```python
from build123d import *

# Parameters (mm, degrees)
SKETCH1_W                = 762
SKETCH1_H                = 457.2
BOSS_EXTRUDE1_DEPTH      = 177.8
SKETCH2_W                = 749.3
SKETCH2_H                = 444.5
CUT_EXTRUDE1_DEPTH       = 171.45
SKETCH4_W                = 758.825
SKETCH4_H                = 454.025
SKETCH4_W_2              = 752.475
SKETCH4_H_2              = 447.675
CUT_EXTRUDE3_DEPTH       = 3.175
SKETCH5_W                = 762
SKETCH5_H                = 12.7
BOSS_EXTRUDE2_DEPTH      = 177.8
BOSS_EXTRUDE2_DEPTH_BACK = 38.1
SKETCH7_R                = 6.35
BOSS_EXTRUDE3_DEPTH      = 762
SKETCH8_W                = 12.7
SKETCH8_H                = 38.1
CUT_EXTRUDE4_DEPTH       = 202.692


with BuildPart() as part:
    # Sketch1 → Boss-Extrude1 (new body)
    with BuildSketch(Plane(origin=(0, 0, 0), x_dir=(1, 0, 0), z_dir=(0, 1, 0))):
        Rectangle(SKETCH1_W, SKETCH1_H)
    extrude(amount=BOSS_EXTRUDE1_DEPTH)

    # Sketch2 → Cut-Extrude1 (cut)
    with BuildSketch(Plane.XZ):
        Rectangle(SKETCH2_W, SKETCH2_H)
    extrude(amount=-CUT_EXTRUDE1_DEPTH, mode=Mode.SUBTRACT)

    # Sketch4 → Cut-Extrude3 (cut)
    with BuildSketch(Plane.XZ):
        Rectangle(SKETCH4_W, SKETCH4_H)
        Rectangle(SKETCH4_W_2, SKETCH4_H_2, mode=Mode.SUBTRACT)
    extrude(amount=-CUT_EXTRUDE3_DEPTH, mode=Mode.SUBTRACT)

    # Sketch5 → Boss-Extrude2 (add, two sides)
    with BuildSketch(Plane(origin=(0, 0, 0), x_dir=(1, 0, 0), z_dir=(0, 1, 0))) as boss_extrude2_sk:
        with Locations((0, -234.95)):
            Rectangle(SKETCH5_W, SKETCH5_H)
    extrude(amount=BOSS_EXTRUDE2_DEPTH)
    extrude(boss_extrude2_sk.sketch, amount=-BOSS_EXTRUDE2_DEPTH_BACK)

    # Sketch7 → Boss-Extrude3 (add)
    with BuildSketch(Plane.ZY.offset(381)):
        with BuildLine():
            Line((-238.125, 9.525), (-238.125, 47.625))
            Line((-238.125, 47.625), (-228.6, 47.625))
            Line((-228.6, 47.625), (-228.6, 0))
            ThreePointArc((-228.6, 0), (-244.860192091, -6.735192091), (-238.125, 9.525))
        make_face()
        with Locations((-238.125, 0)):
            Circle(SKETCH7_R, mode=Mode.SUBTRACT)
    extrude(amount=-BOSS_EXTRUDE3_DEPTH)

    # Sketch8 → Cut-Extrude4 (cut)
    with BuildSketch(Plane(origin=(0, 177.8, 0), x_dir=(1, 0, 0), z_dir=(0, 1, 0))):
        Polygon((-120.65, 266.7), (-133.35, 266.7), (-133.35, 228.6), (-120.65, 228.6), (120.65, 228.6), (133.35, 228.6), (133.35, 266.7), (120.65, 266.7), align=None)
        with Locations((-152.4, 247.65)):
            Rectangle(SKETCH8_W, SKETCH8_H)
        Polygon((-247.65, 228.6), (-260.35, 228.6), (-381, 228.6), (-381, 266.7), (-260.35, 266.7), (-247.65, 266.7), align=None)
        with Locations((-177.8, 247.65)):
            Rectangle(SKETCH8_W, SKETCH8_H)
        with Locations((-228.6, 247.65)):
            Rectangle(SKETCH8_W, SKETCH8_H)
        with Locations((-203.2, 247.65)):
            Rectangle(SKETCH8_W, SKETCH8_H)
        with Locations((152.4, 247.65)):
            Rectangle(SKETCH8_W, SKETCH8_H)
        with Locations((177.8, 247.65)):
            Rectangle(SKETCH8_W, SKETCH8_H)
        with Locations((203.2, 247.65)):
            Rectangle(SKETCH8_W, SKETCH8_H)
        with Locations((228.6, 247.65)):
            Rectangle(SKETCH8_W, SKETCH8_H)
        Polygon((247.65, 266.7), (247.65, 228.6), (260.35, 228.6), (381, 228.6), (381, 266.7), (260.35, 266.7), align=None)
    extrude(amount=-CUT_EXTRUDE4_DEPTH, mode=Mode.SUBTRACT)


solid = part.part
```
Input: part model. Units: mm. Frame: model coordinates. A direction names the side the tool comes from. Round coordinates to 2 decimals unless told otherwise and drop trailing zeros. Loops run counter-clockwise (first coordinate to the right, second up) from the corner with the lowest first, then second, coordinate; pieces in that order, holes last. Notation, with made-up numbers: M 42.5,36 L 89.5,36 A12 ccw 89.5,43 Z; hole C 39,30.25 d2. An arc over 180 degrees is marked long. Answer in a Markdown table with one row per item. Add a question column.
1. Ray query, probe 1 along X at (y, z) = (111, -42); probe 2 along Z at (x, y) = (33, 148); probe 3 along Y at (x, z) = (228, -17). Return the intervals inside material, ascending.
2. Set-up query: faces 5 (the face through (-215.989, -6.954, -244.634)), 6 (the face through (171.45, 19, -236)), 7 (the face through (-5, 85, -222.25)). Return all of +Z, -Z, +X, -X, +Y, -Y with unobstructed straight access to the full face (end or side cutting, diameter ignored); none if empty.
3. Mould query, pull axis X, two halves, no side actions, for faces 1 (the face through (-5, 85, 222.25)), 2 (the face through (-196.85, 19, -236)), 3 (the face through (247.65, 19, -236)), 4 (the face through (190.411, -6.954, -244.634)). Classes: released by +X, released by -X, zero draft, split by the parting line, or undercut.
4. Section A-A (y = 129). Output: boundary loops of the cut face in (x, z), and give its area (3 significant figures).
5. Contact query for flat-ended pins moving along their axis: pin 1 (14 mm diameter, centred on x = 192, y = 23, fed in from -Z) (3 decimals); pin 2 (1 mm diameter, centred on x = 83, y = 38.5, fed in from -Z); pin 3 (1 mm diameter, centred on x = 113.5, y = -9, fed in from -Z). Output: stop coordinate, or through.
Values follow:
| question | item | result |
|---|---|---|
| 1 | probe 1 | -381 to -374.65, 374.65 to 381 |
| 1 | probe 2 | -228.6 to -222.25, 222.25 to 241.3 |
| 1 | probe 3 | 171.45 to 177.8 |
| 2 | face 5 | +X, -X |
| 2 | face 6 | -Z, +Y, -Y |
| 2 | face 7 | -Y |
| 3 | face 1 | undercut |
| 3 | face 2 | undercut |
| 3 | face 3 | released by +X |
| 3 | face 4 | zero draft |
| 4 | outline | M -381,-228.6 L 381,-228.6 L 381,241.3 L -381,241.3 Z; hole M -374.65,-222.25 L 374.65,-222.25 L 374.65,222.25 L -374.65,222.25 Z |
| 4 | area | 25,000 mm^2 |
| 5 | pin 1 | z = -238.125 |
| 5 | pin 2 | z = -228.6 |
| 5 | pin 3 | z = 228.6 |
